```python
from build123d import *

# Parameters (mm, degrees)
SKETCH2_R           = 8.5
BOSS_EXTRUDE1_DEPTH = 13
SKETCH4_W           = 8
SKETCH4_H           = 6
BOSS_EXTRUDE2_DEPTH = 150
BOSS_EXTRUDE2_DRAFT = -1
SKETCH6_R           = 3
BOSS_EXTRUDE3_DEPTH = 120
SKETCH7_R           = 3
BOSS_EXTRUDE4_DEPTH = 120
CUT_EXTRUDE2_REACH  = 157.776
SKETCH8_R           = 3.15
CUT_EXTRUDE3_REACH  = 157.784
CUT_EXTRUDE6_REACH  = 158.041
SKETCH12_W          = 10
SKETCH12_H          = 2.051798714
CUT_EXTRUDE7_REACH  = 157.784
SKETCH13_W          = 43.706918827
SKETCH13_H          = 28.028328295
SKETCH14_W          = 10
SKETCH14_H          = 13.868841859
CUT_EXTRUDE8_DEPTH  = 2
CUT_EXTRUDE9_REACH  = 118.001
SKETCH15_R          = 1.5
SKETCH16_R          = 1.55
CUT_EXTRUDE10_DEPTH = 10


with BuildPart() as part:
    # Sketch2 → Boss-Extrude1 (new body)
    with BuildSketch(Plane.XY):
        with Locations(Location((0, 0, 0), (0, 0, 180))):
            Circle(SKETCH2_R)
    extrude(amount=BOSS_EXTRUDE1_DEPTH)


with BuildPart() as boss_extrude2_tool:
    # Sketch4 → Boss-Extrude2 (with draft: the straight prism first)
    with BuildSketch(Plane(origin=(5, 0, 0), x_dir=(0, 0, -1), z_dir=(1, 0, 0))):
        with Locations((-6.752185146, -0.034660359)):
            Rectangle(SKETCH4_W, SKETCH4_H)
    extrude(amount=BOSS_EXTRUDE2_DEPTH)
    # Boss-Extrude2: the draft: its side faces are tilted about the plane it starts from
    boss_extrude2_sides = [boss_extrude2_tool.faces().sort_by_distance(p)[0] for p in [
        (80, -0.034660359, 10.752185146),
        (80, -3.034660359, 6.752185146),
        (80, -0.034660359, 2.752185146),
        (80, 2.965339641, 6.752185146),
    ]]
    draft(boss_extrude2_sides, Plane(origin=(5, 0, 0), x_dir=(0, 0, -1), z_dir=(1, 0, 0)), BOSS_EXTRUDE2_DRAFT)


with BuildPart() as part_1:
    add(part.part)

    # Boss-Extrude2: add boss_extrude2_tool
    add(boss_extrude2_tool.part)

    # Sketch6 → Boss-Extrude3 (add)
    with BuildSketch(Plane(origin=(0, 0, 0), x_dir=(0, 0, 1), z_dir=(-0.999390827019096, 0.034899496702494044, 0))):
        with Locations((6.68193283, 5.483107785)):
            Circle(SKETCH6_R)
    extrude(amount=-BOSS_EXTRUDE3_DEPTH)

    # Sketch7 → Boss-Extrude4 (add)
    with BuildSketch(Plane(origin=(0, 0, 0), x_dir=(0, 0, 1), z_dir=(0.9993908270190958, 0.034899496702501046, 0))):
        with Locations((6.315850074, 5.431762479)):
            Circle(SKETCH7_R)
    extrude(amount=BOSS_EXTRUDE4_DEPTH)

    # Sketch8 → Cut-Extrude2 (cut, up to next)
    with BuildSketch(Plane.XY.offset(13), mode=Mode.PRIVATE) as cut_extrude2_sk1:
        Circle(SKETCH8_R)
    cut_extrude2_tool1 = extrude(cut_extrude2_sk1.sketch, amount=-CUT_EXTRUDE2_REACH, mode=Mode.PRIVATE) & part_1.part
    add(cut_extrude2_tool1.solids().sort_by_distance((0, 0, 13))[0], mode=Mode.SUBTRACT)

    # Sketch9 → Cut-Extrude3 (cut, up to next)
    with BuildSketch(Plane(origin=(-0.186099993, 0, 10.661661434), x_dir=(0.9998476951563913, 0, 0.01745240643728355), z_dir=(-0.01745240643728355, 0, 0.9998476951563913)), mode=Mode.PRIVATE) as cut_extrude3_sk1:
        Polygon((13.337744906, 3.107591674), (30.337744906, 3.404282584), (30.337744906, 5.218463822), (13.337744906, 5.218463822), align=None)
    cut_extrude3_tool1 = extrude(cut_extrude3_sk1.sketch, amount=-CUT_EXTRUDE3_REACH, mode=Mode.PRIVATE) & part_1.part
    # Sketch9 → Cut-Extrude3 (cut, up to next)
    with BuildSketch(Plane(origin=(-0.186099993, 0, 10.661661434), x_dir=(0.9998476951563913, 0, 0.01745240643728355), z_dir=(-0.01745240643728355, 0, 0.9998476951563913)), mode=Mode.PRIVATE) as cut_extrude3_sk2:
        Polygon((43.018729252, 3.625596277), (60.018729252, 3.922287186), (60.018729252, 5.218463822), (43.018729252, 5.218463822), align=None)
    cut_extrude3_tool2 = extrude(cut_extrude3_sk2.sketch, amount=-CUT_EXTRUDE3_REACH, mode=Mode.PRIVATE) & part_1.part
    # Sketch9 → Cut-Extrude3 (cut, up to next)
    with BuildSketch(Plane(origin=(-0.186099993, 0, 10.661661434), x_dir=(0.9998476951563913, 0, 0.01745240643728355), z_dir=(-0.01745240643728355, 0, 0.9998476951563913)), mode=Mode.PRIVATE) as cut_extrude3_sk3:
        Polygon((13.624548626, -3.181917807), (30.624548626, -3.478608716), (30.624548626, -5.320643976), (13.624548626, -5.320643976), align=None)
    cut_extrude3_tool3 = extrude(cut_extrude3_sk3.sketch, amount=-CUT_EXTRUDE3_REACH, mode=Mode.PRIVATE) & part_1.part
    # Sketch9 → Cut-Extrude3 (cut, up to next)
    with BuildSketch(Plane(origin=(-0.186099993, 0, 10.661661434), x_dir=(0.9998476951563913, 0, 0.01745240643728355), z_dir=(-0.01745240643728355, 0, 0.9998476951563913)), mode=Mode.PRIVATE) as cut_extrude3_sk4:
        Polygon((43.018729252, -3.694916994), (60.018729252, -3.991607903), (60.018729252, -5.320643976), (43.018729252, -5.320643976), align=None)
    cut_extrude3_tool4 = extrude(cut_extrude3_sk4.sketch, amount=-CUT_EXTRUDE3_REACH, mode=Mode.PRIVATE) & part_1.part
    add(cut_extrude3_tool1.solids().sort_by_distance((21.434183, 4.235332, 11.039045))[0], mode=Mode.SUBTRACT)
    add(cut_extrude3_tool2.solids().sort_by_distance((51.033857, 4.493664, 11.555709))[0], mode=Mode.SUBTRACT)
    add(cut_extrude3_tool3.solids().sort_by_distance((21.723939, -4.323611, 11.044103))[0], mode=Mode.SUBTRACT)
    add(cut_extrude3_tool4.solids().sort_by_distance((51.040328, -4.579471, 11.555822))[0], mode=Mode.SUBTRACT)

    # Cut-Extrude6: up to this plane
    cut_extrude6_end = Plane(origin=(5, -3.034660359, 10.752185146), z_dir=(-0.01745240643728355, -0.9998476951563913, 0))
    # Sketch12 → Cut-Extrude6 (cut, up to the surface)
    with BuildSketch(Plane(origin=(-0.050221498, 2.877187697, 0), x_dir=(0.9998476951563913, 0.01745240643728355, 0), z_dir=(-0.01745240643728355, 0.9998476951563913, 0)), mode=Mode.PRIVATE) as cut_extrude6_sk1:
        with Locations((141.40635612, -10.3349379)):
            Rectangle(SKETCH12_W, SKETCH12_H)
    cut_extrude6_tool1 = split(extrude(cut_extrude6_sk1.sketch, amount=-CUT_EXTRUDE6_REACH, mode=Mode.PRIVATE), bisect_by=cut_extrude6_end, keep=Keep.BOTH, mode=Mode.PRIVATE)
    add(cut_extrude6_tool1.solids().sort_by_distance((141.334598, 5.345069, 10.334938))[0], mode=Mode.SUBTRACT)

    # Cut-Extrude7: up to this plane
    cut_extrude7_end = Plane(origin=(5, 2.965339641, 2.752185146), z_dir=(-0.01745240643728355, 0, -0.9998476951563913))
    # Sketch13 → Cut-Extrude7 (cut, up to the surface)
    with BuildSketch(Plane(origin=(-0.186099993, 0, 10.661661434), x_dir=(0.9998476951563913, 0, 0.01745240643728355), z_dir=(-0.01745240643728355, 0, 0.9998476951563913)), mode=Mode.PRIVATE) as cut_extrude7_sk1:
        with Locations((137.063198602, -4.734636569)):
            Rectangle(SKETCH13_W, SKETCH13_H)
    cut_extrude7_tool1 = split(extrude(cut_extrude7_sk1.sketch, amount=-CUT_EXTRUDE7_REACH, mode=Mode.PRIVATE), bisect_by=cut_extrude7_end, keep=Keep.BOTH, mode=Mode.PRIVATE)
    add(cut_extrude7_tool1.solids().sort_by_distance((136.856223, -4.734637, 13.053744))[0], mode=Mode.SUBTRACT)

    # Sketch14 → Cut-Extrude8 (cut)
    with BuildSketch(Plane(origin=(-0.186099993, 0, 10.661661434), x_dir=(0.9998476951563913, 0, 0.01745240643728355), z_dir=(-0.01745240643728355, 0, 0.9998476951563913))):
        with Locations((110.243167646, 0.778255403)):
            Rectangle(SKETCH14_W, SKETCH14_H)
    extrude(amount=-CUT_EXTRUDE8_DEPTH, mode=Mode.SUBTRACT)

    # Cut-Extrude9: up to this plane
    cut_extrude9_end = Plane(origin=(5, 2.965339641, 2.752185146), z_dir=(-0.01745240643728355, 0, -0.9998476951563913))
    # Sketch15 → Cut-Extrude9 (cut, up to the surface)
    with BuildSketch(Plane(origin=(-0.15119518, 0, 8.661966044), x_dir=(0.9998476951563913, 0, 0.017452406437283588), z_dir=(-0.017452406437283588, 0, 0.9998476951563913)), mode=Mode.PRIVATE) as cut_extrude9_sk1:
        with Locations((110.220200994, 2.297708244)):
            Circle(SKETCH15_R)
    cut_extrude9_tool1 = split(extrude(cut_extrude9_sk1.sketch, amount=-CUT_EXTRUDE9_REACH, mode=Mode.PRIVATE), bisect_by=cut_extrude9_end, keep=Keep.BOTH, mode=Mode.PRIVATE)
    add(cut_extrude9_tool1.solids().sort_by_distance((110.052219, 2.297708, 10.585574))[0], mode=Mode.SUBTRACT)
    # Sketch15 → Cut-Extrude9 (cut, up to the surface)
    with BuildSketch(Plane(origin=(-0.15119518, 0, 8.661966044), x_dir=(0.9998476951563913, 0, 0.017452406437283588), z_dir=(-0.017452406437283588, 0, 0.9998476951563913)), mode=Mode.PRIVATE) as cut_extrude9_sk2:
        with Locations((110.209739188, -2.702291756)):
            Circle(SKETCH15_R)
    cut_extrude9_tool2 = split(extrude(cut_extrude9_sk2.sketch, amount=-CUT_EXTRUDE9_REACH, mode=Mode.PRIVATE), bisect_by=cut_extrude9_end, keep=Keep.BOTH, mode=Mode.PRIVATE)
    add(cut_extrude9_tool2.solids().sort_by_distance((110.041759, -2.702292, 10.585391))[0], mode=Mode.SUBTRACT)

    # Sketch16 → Cut-Extrude10 (cut, symmetric)
    with BuildSketch(Plane(origin=(0, 0, 0), x_dir=(1, 0, 0), z_dir=(0, 1, 0))):
        with Locations(Location((-0.73595313, -5.950294761, 0), (0, 0, 270))):
            Circle(SKETCH16_R)
    extrude(amount=CUT_EXTRUDE10_DEPTH, both=True, mode=Mode.SUBTRACT)


solid = part_1.part
```
The listing builds one solid part. Answer for the finished solid, in the listing's coordinates (mm). Round coordinates to 2 decimals unless told otherwise and drop trailing zeros. Put each result on its own line as item: value. Start each with the question number.
(1) Given P1, Ø1, axis at y = -5, z = 11, coming from the +X side; P2, Ø4, axis at x = 38, z = 3, coming from the -Y side; P3, Ø4, axis at x = 72, y = -0.5, coming from the +Z side, each flat-ended and moving along its own axis, determine where each tip first touches the part or whether it passes through.
(2) Determine the mould class of faces 1 (the flat face through (-4, 0, 0)), 2 (the flat face through (22, 5.218, 7)) for opening direction X: released by +X, released by -X, zero draft, split by the parting line, or undercut.
(3) Find section A-A (x = 26.5). State how many separate pieces and enclosed holes the cut face has, plus the area to 3 significant figures.
(4) Straight lines are drawn through the part: probe 1 along Y at (x, z) = (26.5, 8.5); probe 2 along X at (y, z) = (2.75, 5); probe 3 along Y at (x, z) = (21, 4). For each, find the intervals that lie inside material, in ascending order. Write a range as from..to.
Reply:
1. P1: x = 115.04
1. P2: y = -6.81
1. P3: z = 11.96
2. face 1: zero draft
2. face 2: undercut
3. separate pieces: 3
3. enclosed holes: 0
3. area: 78.6 mm^2
4. probe 1: -6.57..-5.32, -3.41..3.34, 5.22..6.95
4. probe 2: -8.04..-1.96, 1.54..108.72, 111.58..115.14
4. probe 3: -6.61..-5.32, -3.31..3.24, 5.22..6.1
